Could you check a few things on this model? Use its own coordinates, in mm. Face numbers are marked on the shaded views. Give positions to 0.01 mm unless a question says otherwise; leave off trailing zeros. Loops run counter-clockwise (first coordinate to the right, second up) from the corner with the lowest first, then second, coordinate; pieces in that order, holes last.
1. For P1, Ø4, axis at y = 7.5, z = -2.5, coming from the +X side; P2, Ø1.5, axis at x = 6.5, y = 7, coming from the -Z side; P3, Ø2, axis at x = 4, z = -3, coming from the -Y side; P4, Ø6, axis at x = 0, y = 0, coming from the -Z side, each with a flat end and sliding along its axis, tell me the tip position at first contact or that it passes through.
2. Imagine slicing it at A-A (y = 0). List the corners of the cut face in (x, z) for me, plus the area to 3 significant figures.
3. I need wall thicknesses on line 1 along Y through (x, z) = (0, -5.5); line 2 along X through (y, z) = (-8.5, -6.5); line 3 along Z through (x, y) = (-4, -6.5). Which ranges of each line are inside material? Lowest first, please.
4. Thinking about a two-plate mould opening in Y: for the marked faces 1, 2 and 3, which applies, +Y half, -Y half, draft (parallel to the pull), parting line (faces both ways), or undercut?
5. Imagine slicing it at C-C (z = -2.5). List the corners of the cut face in (x, y) for me (1 decimal), plus the area to 3 significant figures.
6. Imagine slicing it at D-D (z = -10). List the corners of the cut face in (x, y) for me, plus the area to 3 significant figures.
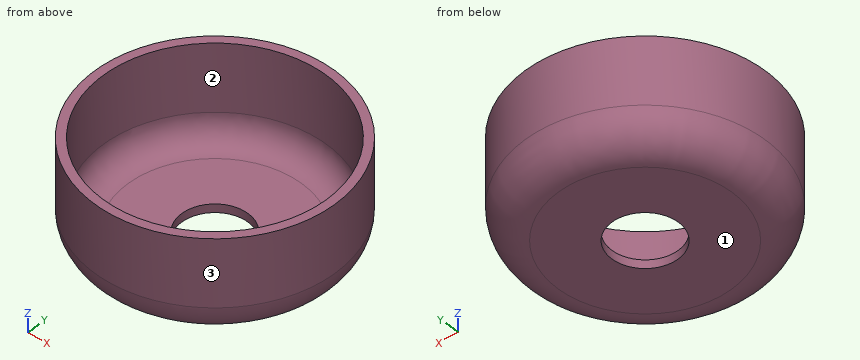
```python
from build123d import *

# Parameters (mm, degrees)
CUT_EXTRUDE1_DEPTH      = 21.261822212
CUT_EXTRUDE1_DEPTH_BACK = 21.261822212
SKETCH2_W               = 23.9014
SKETCH2_H               = 12.352
SKETCH3_R               = 3.3
CUT_EXTRUDE2_DEPTH      = 20.224386664


with BuildPart() as part:
    # Sketch1 → Revolve1 (revolve)
    with BuildSketch(Plane(origin=(0, 0, 0), x_dir=(0, 0, -1), z_dir=(1, 0, 0)), mode=Mode.PRIVATE) as revolve1_sk:
        with BuildLine():
            Line((-11.176, 11.9507), (-11.176, 11.1125))
            Line((-11.176, 11.1125), (7.874, 11.1125))
            ThreePointArc((7.874, 11.1125), (9.616169687, 10.390869687), (10.3378, 8.6487))
            Line((10.3378, 8.6487), (10.3378, 0))
            Line((10.3378, 0), (11.176, 0))
            Line((11.176, 0), (11.176, 8.6487))
            ThreePointArc((11.176, 8.6487), (10.208866591, 10.983566591), (7.874, 11.9507))
            Line((7.874, 11.9507), (-11.176, 11.9507))
        make_face()
    revolve(revolve1_sk.sketch.rotate(Axis((0, 0, 11.176), (0, 0, -1)), 90), axis=Axis((0, 0, 11.176), (0, 0, -1)))

    # Sketch2 → Cut-Extrude1 (cut, two sides: drawn at the far end of the back side and taken through both)
    with BuildSketch(Plane(origin=(0, 0, 0), x_dir=(1, 0, 0), z_dir=(0, 1, 0)).offset(-CUT_EXTRUDE1_DEPTH_BACK)):
        with Locations((0, -5)):
            Rectangle(SKETCH2_W, SKETCH2_H)
    extrude(amount=CUT_EXTRUDE1_DEPTH + CUT_EXTRUDE1_DEPTH_BACK, mode=Mode.SUBTRACT)

    # Sketch3 → Cut-Extrude2 (cut, through all)
    with BuildSketch(Plane.XY.offset(-10.3378)):
        Circle(SKETCH3_R)
    extrude(amount=-CUT_EXTRUDE2_DEPTH, mode=Mode.SUBTRACT)


solid = part.part
```
Derived:
1. P1: stops at x = 10.61
1. P2: stops at z = -11.17
1. P3: stops at y = -11.57
1. P4: passes through
2. outline: (-11.95, -7.87) arc R3.3 ccw to (-8.65, -11.18) - (-3.3, -11.18) - (-3.3, -10.34) - (-8.65, -10.34) arc R2.46 cw to (-11.11, -7.87) - (-11.11, -1.18) - (-11.95, -1.18) - close; (3.3, -11.18) - (8.65, -11.18) arc R3.3 ccw to (11.95, -7.87) - (11.95, -1.18) - (11.11, -1.18) - (11.11, -7.87) arc R2.46 cw to (8.65, -10.34) - (3.3, -10.34) - close
2. area: 27.8 mm2
3. line 1: y = -11.95 to -11.11, 11.11 to 11.95
3. line 2: x = -8.4 to -7.16, 7.16 to 8.4
3. line 3: z = -11.18 to -10.34
4. face 1: draft
4. face 2: undercut
4. face 3: parting line
5. outline: circle Ø23.9 at (0, 0); hole circle Ø22.2 at (0, 0)
5. area: 60.7 mm2
6. outline: circle Ø22.35 at (0, 0); hole circle Ø19.79 at (0, 0)
6. area: 84.8 mm2
